from build123d import *

# Parameters (mm, degrees)
F0_R     = 2.787797
F0_R_2   = 2.613336
F1_DEPTH = 3
F2_R     = 1.110605
F2_R_2   = 1.099003
F3_DEPTH = 25


with BuildPart() as f1:
    # F0 (on Front) → F1 (new body)
    with BuildSketch(Plane.XZ):
        with BuildLine():
            Line((15.031415, 7.53661), (-15.120215, 7.53661))
            ThreePointArc((-15.120215, 7.53661), (-18.655749, 6.072144), (-20.120215, 2.53661))
            Line((-20.120215, 2.53661), (-20.120215, -2.491496))
            ThreePointArc((-20.120215, -2.491496), (-18.655749, -6.02703), (-15.120215, -7.491496))
            Line((-15.120215, -7.491496), (15.031415, -7.491496))
            ThreePointArc((15.031415, -7.491496), (18.566949, -6.02703), (20.031415, -2.491496))
            Line((20.031415, -2.491496), (20.031415, 2.53661))
            ThreePointArc((20.031415, 2.53661), (18.566949, 6.072144), (15.031415, 7.53661))
        make_face()
        with Locations((-13.596544, 0)):
            Circle(F0_R, mode=Mode.SUBTRACT)
        with Locations((-2.956751, 0)):
            Circle(F0_R_2, mode=Mode.SUBTRACT)
    extrude(amount=F1_DEPTH)

    # F2 (on face) → F3 (cut)
    with BuildSketch(Plane(origin=(0, 0, 0), x_dir=(-1, 0, 0), z_dir=(0, 1, 0))):
        with Locations((-12.780892, 4.825667)):
            Circle(F2_R)
        with Locations((-12.780892, -4.649186)):
            Circle(F2_R_2)
    extrude(amount=-F3_DEPTH, mode=Mode.SUBTRACT)


solid = f1.part
Read the model definition and answer for the solid it produces. Units are mm, in the model's axes. Round coordinates to 2 decimals unless told otherwise and drop trailing zeros. Write each loop counter-clockwise with the first axis right and the second up, starting at its lowest first coordinate (ties: lowest second). Pieces come first, ordered by that corner, then holes. Notation, with made-up numbers: (4.25, 40.5) - (47.25, 40.5) arc R10 ccw to (47.25, 53.5) - close; hole circle Ø9 at (72, 20). An arc over 180 degrees is marked (long way). Use a Markdown table: item, result.
(1) The part is cut by section B-B (x = 12.5). Write down the section's boundary in (y, z).
Reported:
| item | result |
|---|---|
| outline | (-3, -7.49) - (0, -7.49) - (0, -5.71) - (-3, -5.71) - close; (-3, -3.59) - (0, -3.59) - (0, 3.75) - (-3, 3.75) - close; (-3, 5.9) - (0, 5.9) - (0, 7.54) - (-3, 7.54) - close |
(2) The mould has two halves that part along Z. Classify faces 1 (the cylindrical face through (-18.62, -1.48, 6.11)), 2 (the cylindrical face through (11.766, -1.479, -5.07)), 3 (the flat face through (-20.12, -1, 0)), 4 (the cylindrical face through (18.528, -1.479, -6.066)): released by +Z, released by -Z, zero draft, split by the parting line, or undercut.
Reported:
| item | result |
|---|---|
| face 1 | released by +Z |
| face 2 | undercut |
| face 3 | zero draft |
| face 4 | released by -Z |
(3) Straight lines are drawn through the part: line 1 along X through (y, z) = (-1.95, -2); line 2 along X through (y, z) = (-1.45, -0.75); line 3 along Z through (x, y) = (12.5, -1.25). For each, find the intervals that lie inside material, in ascending order. Write a range as [from, to].
Reported:
| item | result |
|---|---|
| line 1 | [-20.12, -15.54], [-11.65, -4.64], [-1.27, 20.03] |
| line 2 | [-20.12, -16.28], [-10.91, -5.46], [-0.45, 20.03] |
| line 3 | [-7.49, -5.71], [-3.59, 3.75], [5.9, 7.54] |
(4) The part is cut by section D-D (x = 17). Write down the section's boundary in (y, z).
Reported:
| item | result |
|---|---|
| outline | (-3, -7.09) - (0, -7.09) - (0, 7.13) - (-3, 7.13) - close |
(5) The part is cut by section C-C (y = -2.45). Write down the section's boundary in (x, z), then the cut area to 3 significant figures.
Reported:
| item | result |
|---|---|
| outline | (-20.12, -2.49) arc R5 ccw to (-15.12, -7.49) - (15.03, -7.49) arc R5 ccw to (20.03, -2.49) - (20.03, 2.54) arc R5 ccw to (15.03, 7.54) - (-15.12, 7.54) arc R5 ccw to (-20.12, 2.54) - close; hole circle Ø5.58 at (-13.6, 0); hole circle Ø5.23 at (-2.96, 0); hole circle Ø2.22 at (12.78, 4.83); hole circle Ø2.2 at (12.78, -4.65) |
| area | 528 mm2 |
(6) This flat-tipped pin is pushed along its axis until it touches: pin 1 Ø5 at (x, z) = (-13.6, 0) entering from +Y. Where does it stop, or does it pass through?
Reported:
| item | result |
|---|---|
| pin 1 | through |
(7) The part is cut by section A-A (z = 0). Write down the section's boundary in (x, y), then the cut area to 3 significant figures.
Reported:
| item | result |
|---|---|
| outline | (-20.12, -3) - (-16.38, -3) - (-16.38, 0) - (-20.12, 0) - close; (-10.81, -3) - (-5.57, -3) - (-5.57, 0) - (-10.81, 0) - close; (-0.34, -3) - (20.03, -3) - (20.03, 0) - (-0.34, 0) - close |
| area | 88.0 mm2 |
